Here's how the part is built. I have some questions about the finished solid (model axes, mm). Face numbers are marked on the shaded views. A direction names the side the tool comes from. Coordinates: 2 decimals unless noted, no trailing zeros. Order: outer loops, then holes, each group sorted by start corner. A loop starts at its lowest first (then second) coordinate and runs counter-clockwise, first axis right, second up. Notation, with made-up numbers: (44.5, 27.5) - (52.5, 27.5) arc R24 ccw to (52.5, 43.5) - close; hole circle Ø7 at (-36.75, -10.75). An arc over 180 degrees is marked (long way). Answer as CSV lines item,"result". Start each with the question number.
Q1. I need wall thicknesses on line 1 (Z direction, x = -1.25, y = 6); line 2 (Y direction, x = -0.5, z = -0.25); line 3 (Y direction, x = -0.25, z = -8.25). Which ranges of each line are inside material? Lowest first, please.
Q2. Suppose I cut it at D-D (z = -7.25). Please give me the cut outline in (x, y).
Q3. For the marked faces 4 and 5, which set-ups out of +Z, -Z, +X, -X, +Y, -Y let a thin tool reach every point of the face, with its end or its side?
Q4. Suppose I cut it at C-C (z = 1.75). Please give me the cut outline in (x, y), then the cut area to 3 significant figures.
Q5. Thinking about a two-plate mould opening in X: for the marked faces 1, 2 and 3, which applies, released by +X, released by -X, zero draft, split by the parting line, or undercut?
Q6. Suppose I cut it at B-B (y = 0). Count the separate pieces of the cut face and the enclosed holes in it, then the cut area to 3 significant figures.
Q7. For pin 1 Ø1.5 at (x, y) = (-1.5, 5.5) entering from +Z; pin 2 Ø0.6 at (x, z) = (2.5, -12) entering from +Y; pin 3 Ø1 at (x, z) = (5.5, -10.5) entering from +Y; pin 4 Ø1.5 at (y, z) = (-0.5, -11.5) entering from +X, each with a flat end and sliding along its axis, tell me the tip position at first contact or that it passes through.
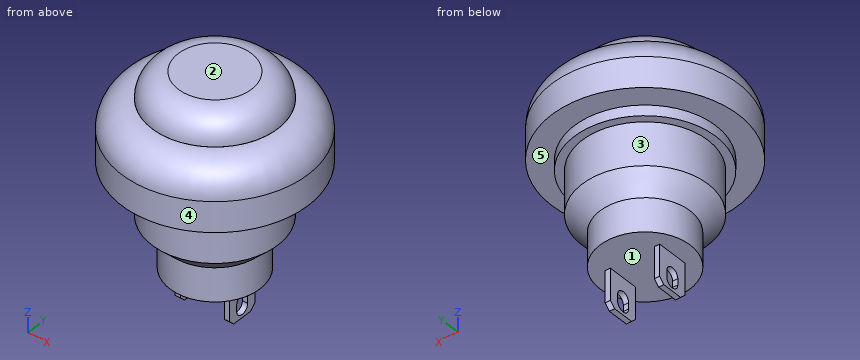
from build123d import *

# Parameters (mm, degrees)
SKETCH_1_R          = 8.9
EXTRUDE_1_DEPTH     = 5.8
FILLET_2_R          = 2.9
SKETCH_2_R          = 6.75
EXTRUDE_2_DEPTH     = 1
SKETCH_3_R          = 6
EXTRUDE_3_DEPTH     = 7.5
SKETCH_4_R          = 4.3
EXTRUDE_4_DEPTH     = 1.5
CHAMFER_1_SIZE      = 3.4
EXTRUDE_5_DEPTH     = 3.5
CUT_EXTRUDE_1_DEPTH = 6.5
CHAMFER_2_SIZE      = 0.5
EXTRUDE_START       = 2.5
SKETCH_7_R          = 6
EXTRUDE_6_DEPTH     = 2.5
FILLET_3_R          = 2.5


# Some blends are built 0.0001 mm under size
with BuildPart() as part:
    # 草图1 → 凸台-拉伸1 (new body)
    with BuildSketch(Plane.XY):
        Circle(SKETCH_1_R)
    extrude(amount=EXTRUDE_1_DEPTH)

    # 圆角2
    fillet_2_edges = [part.edges().sort_by_distance(p)[0] for p in [
        (-8.9, 0, 5.8),
    ]]
    fillet(fillet_2_edges, radius=FILLET_2_R)

    # 草图2 → 凸台-拉伸2 (add)
    with BuildSketch(Plane(origin=(0, 0, 0), x_dir=(-1, 0, 0), z_dir=(0, 0, -1))):
        with Locations(Location((0, 0, 0), (0, 0, 180))):
            Circle(SKETCH_2_R)
    extrude(amount=EXTRUDE_2_DEPTH)

    # 草图3 → 凸台-拉伸3 (add)
    with BuildSketch(Plane(origin=(0, 0, -1), x_dir=(-1, 0, 0), z_dir=(0, 0, -1))):
        Circle(SKETCH_3_R)
    extrude(amount=EXTRUDE_3_DEPTH)

    # 草图4 → 凸台-拉伸4 (add)
    with BuildSketch(Plane(origin=(0, 0, -8.5), x_dir=(-1, 0, 0), z_dir=(0, 0, -1))):
        Circle(SKETCH_4_R)
    extrude(amount=EXTRUDE_4_DEPTH)

    # 倒角1
    # the kernel refuses this chamfer: 3.4 mm, written as the material it takes off along each edge
    with BuildSketch(Plane(origin=(0, 0, -8.5), x_dir=(-1, 0, 0), z_dir=(0, -1, 0))) as chamfer_1_piece_1_section:
        Polygon((6, -CHAMFER_1_SIZE), (6 - CHAMFER_1_SIZE, 0), (6, 0), align=None)
    chamfer_1_piece_1 = revolve(axis=Axis((0, 0, -8.5), (0, 0, -1)), mode=Mode.PRIVATE)
    chamfer_1_piece_1 = chamfer_1_piece_1 - Plane(origin=(0, 0, -5.94008013), x_dir=(-1, 0, 0), z_dir=(0, 0, 1)) * Cylinder(4.3, 24, mode=Mode.PRIVATE)
    add(chamfer_1_piece_1, mode=Mode.SUBTRACT)

    # 草图5 → 凸台-拉伸5 (add)
    with BuildSketch(Plane(origin=(0, 0, -10), x_dir=(-1, 0, 0), z_dir=(0, 0, -1))):
        Polygon((-2.6, 1.5), (-2.1, 1.5), (-2.1, 0), (-2.1, -1.5), (-2.6, -1.5), align=None)
        Polygon((2.1, 0), (2.1, 1.5), (2.6, 1.5), (2.6, -1.5), (2.1, -1.5), align=None)
    extrude(amount=EXTRUDE_5_DEPTH)

    # 草图6 → 切除-拉伸1 (cut)
    with BuildSketch(Plane.ZY.offset(2.6)):
        with BuildLine():
            Line((-12.55, 0.65), (-11.95, 0.65))
            ThreePointArc((-11.95, 0.65), (-11.3, 0), (-11.95, -0.65))
            Line((-11.95, -0.65), (-12.55, -0.65))
            ThreePointArc((-12.55, -0.65), (-13.2, 0), (-12.55, 0.65))
        make_face()
    extrude(amount=-CUT_EXTRUDE_1_DEPTH, mode=Mode.SUBTRACT)

    # 倒角2
    chamfer_2_edges = [part.edges().sort_by_distance(p)[0] for p in [
        (-2.35, -1.5, -13.5),
        (-2.35, 1.5, -13.5),
        (2.35, -1.5, -13.5),
        (2.35, 1.5, -13.5),
    ]]
    chamfer(chamfer_2_edges, length=CHAMFER_2_SIZE)

    # 草图7 → 凸台-拉伸6 (add)
    with BuildSketch(Plane.XY.offset(5.8).offset(EXTRUDE_START)):
        with Locations(Location((0, 0, 0), (0, 0, 180))):
            Circle(SKETCH_7_R)
    extrude(amount=-EXTRUDE_6_DEPTH)

    # 圆角3
    fillet_3_edges = [part.edges().sort_by_distance(p)[0] for p in [
        (6, 0, 8.3),
    ]]
    fillet(fillet_3_edges, radius=FILLET_3_R - 0.0001)  # a hair under: the kernel refuses the full size


solid = part.part
Here are the results:
1,line 1,"z = -1 to 5.8"
1,line 2,"y = -6.73 to 6.73"
1,line 3,"y = -4.29 to 4.29"
2,outline,"circle Ø8.6 at (0, 0)"
3,face 4,"+Z, -Z"
3,face 5,"-Z"
4,outline,"circle Ø17.8 at (0, 0)"
4,area,"249 mm²"
5,face 1,"undercut"
5,face 2,"zero draft"
5,face 3,"split by the parting line"
6,separate pieces,"3"
6,enclosed holes,"0"
6,area,"236 mm²"
7,pin 1,"stops at z = 7.84"
7,pin 2,"stops at y = 1.5"
7,pin 3,"passes through"
7,pin 4,"stops at x = 2.6"
